Input: dimensioned drawing with shaded views. Units: mm. Origin: part minimum x, y, z. Coordinates: 2 decimals unless noted, no trailing zeros. Order: outer loops, then holes, each group sorted by start corner. A loop starts at its lowest first (then second) coordinate and runs counter-clockwise, first axis right, second up. Notation, with made-up numbers: (0.25, 55.25) - (50.25, 55.25) arc R32 ccw to (50.25, 83.25) - close; hole circle Ø9 at (50.25, -14). An arc over 180 degrees is marked (long way). One line per question, with ' | ' between items. Start each with the question number.
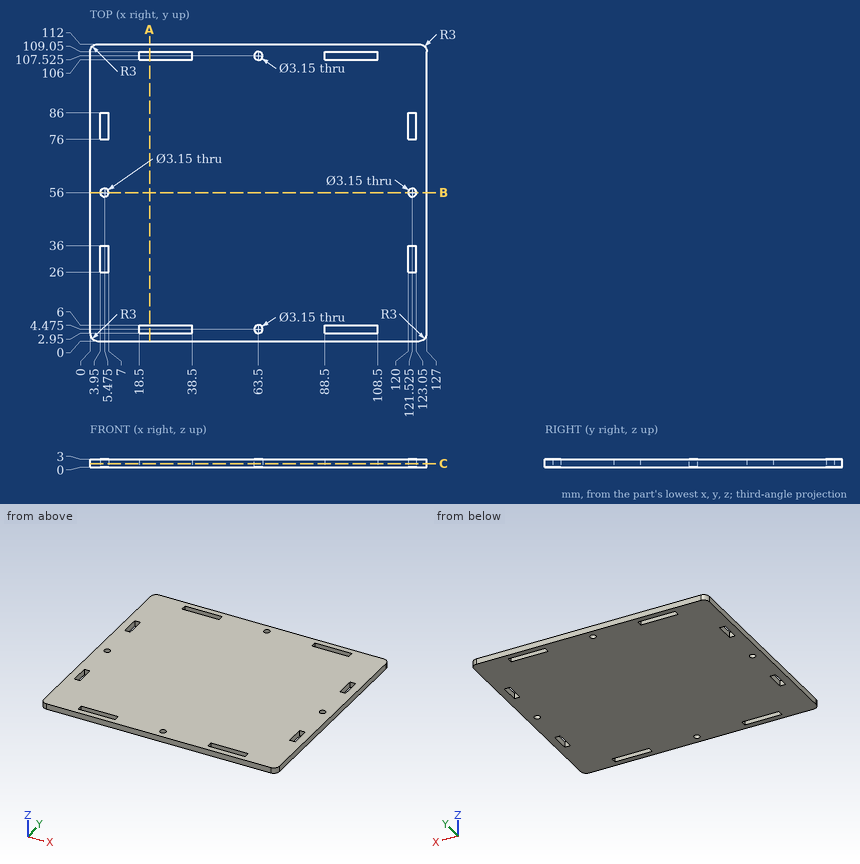
(1) Section B-B (y = 56). Output: boundary loops of the cut face in (x, z).
(2) Section A-A (x = 22.5). Output: boundary loops of the cut face in (y, z).
(3) Section C-C (z = 1.3). State how many separate pieces and enclosed holes the cut face has, then the cut area to 3 significant figures.
(4) Material intervals for line 1 along Y through (x, z) = (63.5, 2.45); line 2 along Y through (x, z) = (100.5, 0.25); line 3 along X through (y, z) = (35.5, 1.95), sorted ascending. Write a range as from..to.
Worked answers:
1) outline: (0, 0) - (3.9, 0) - (3.9, 3) - (0, 3) - close; (7.05, 0) - (119.95, 0) - (119.95, 3) - (7.05, 3) - close; (123.1, 0) - (127, 0) - (127, 3) - (123.1, 3) - close
2) outline: (0, 0) - (2.95, 0) - (2.95, 3) - (0, 3) - close; (6, 0) - (106, 0) - (106, 3) - (6, 3) - close; (109.05, 0) - (112, 0) - (112, 3) - (109.05, 3) - close
3) separate pieces: 1 | enclosed holes: 12 | area: 13,800 mm²
4) line 1: y = 0..2.9, 6.05..105.95, 109.1..112 | line 2: y = 0..2.95, 6..106, 109.05..112 | line 3: x = 0..3.95, 7..120, 123.05..127
